Here's how the part is built. I have some questions about the finished solid (model axes, mm). Coordinates: 2 decimals unless noted, no trailing zeros. Write each loop counter-clockwise with the first axis right and the second up, starting at its lowest first coordinate (ties: lowest second). Pieces come first, ordered by that corner, then holes.
Item 1: I want a section at C-C (x = -0.7). Please give me the cut outline in (y, z), and give its area (3 significant figures).
Item 2: Please list where these lines run through material, in increasing order: line 1 (X direction, y = -3.75, z = 0.35); line 2 (Z direction, x = 0.45, y = -15.75).
Item 3: I want a section at A-A (y = -12.5). Please give me the cut outline in (x, z), and give its area (3 significant figures).
Item 4: I want a section at B-B (z = -1.2). Please give me the cut outline in (x, y).
Autodesk Inventor part; units mm, degrees
ref_plane "YZ Plane" through (0, 0, 0) normal (1, 0, 0) x (0, 1, 0)
ref_plane "XZ Plane" through (0, 0, 0) normal (0, 1, 0) x (-1, 0, 0)
ref_plane "XY Plane" through (0, 0, 0) normal (0, 0, 1) x (1, 0, 0)
sketch "Esquisse1" plane through (0, 0, 0) normal (0, 1, 0) x (-1, 0, 0)
  line L0 (0.3187, 0.4542) -> (-0.3813, 0.4542)
  line L1 (-0.3813, 0.4542) -> (-0.3813, -1.4458)
  line L2 (-0.3813, -1.4458) -> (0.3187, -1.4458)
  line L3 (0.3187, -1.4458) -> (0.3187, 0.4542)
  line L4 (0.9187, -0.8458) -> (-0.9813, -0.8458)
  line L5 (-0.9813, -0.8458) -> (-0.9813, -0.1458)
  line L6 (-0.9813, -0.1458) -> (0.9187, -0.1458)
  line L7 (0.9187, -0.1458) -> (0.9187, -0.8458)
  point P0 (0, 0)
  dimension "d0" = 0.7
  dimension "d1" = 0.7
  dimension "d2" = 1.9
  dimension "d3" = 1.9
  dimension "d4" = 0.6
  dimension "d5" = 0.6
extrude "Extrusion1" add sketch "Esquisse1" against normal blind 20.45
properties part number "Croisillon"
Answer:
1. outline: (-20.45, -0.85) - (0, -0.85) - (0, -0.15) - (-20.45, -0.15) - close
1. area: 14.3 mm2
2. line 1: x = -0.32 to 0.38
2. line 2: z = -0.85 to -0.15
3. outline: (-0.92, -0.85) - (-0.32, -0.85) - (-0.32, -1.45) - (0.38, -1.45) - (0.38, -0.85) - (0.98, -0.85) - (0.98, -0.15) - (0.38, -0.15) - (0.38, 0.45) - (-0.32, 0.45) - (-0.32, -0.15) - (-0.92, -0.15) - close
3. area: 2.17 mm2
4. outline: (-0.32, -20.45) - (0.38, -20.45) - (0.38, 0) - (-0.32, 0) - close
